Part model, mm, in its own coordinate system. Face numbers are marked on the shaded views. Round coordinates to 2 decimals unless told otherwise and drop trailing zeros. Loops run counter-clockwise (first coordinate to the right, second up) from the corner with the lowest first, then second, coordinate; pieces in that order, holes last. Notation, with made-up numbers: M -2,2.25 L 55,2.25 A11 cw 55,20.25 Z; hole C 25.25,78.25 d5. An arc over 180 degrees is marked long. Put each result on its own line as item: value. Start each with the question number.
1) Slice it at D-D on z = -4. Give the cut face in (x, y), then the cut area to 3 significant figures.
2) Probe line 1 along Y through (x, z) = (1.6, 0) (3 decimals); line 2 along Y through (x, z) = (1.9, -1.25) (3 decimals); line 3 along Z through (x, y) = (1.8, 1.75). List the from-to ranges inside material, lowest first.
3) Pull direction Z, two halves, no side cores. Call the marked faces 1, 2 and 3: +Z half, -Z half, draft (parallel to the pull), parting line (faces both ways), or undercut.
4) Slice it at A-A on z = 0. Give the cut face in (x, y) (3 decimals).
5) Slice it at B-B on x = 1.25. Give the cut face in (y, z) (3 decimals), then the cut area to 3 significant figures.
6) Drop a flat-ended pin along its axis: pin 1 Ø1 at (x, y) = (0.5, -3) entering from -Z. Give the stop position or say it passes through.
7) Slice it at C-C on y = 3. Give the cut face in (x, z), then the cut area to 3 significant figures.
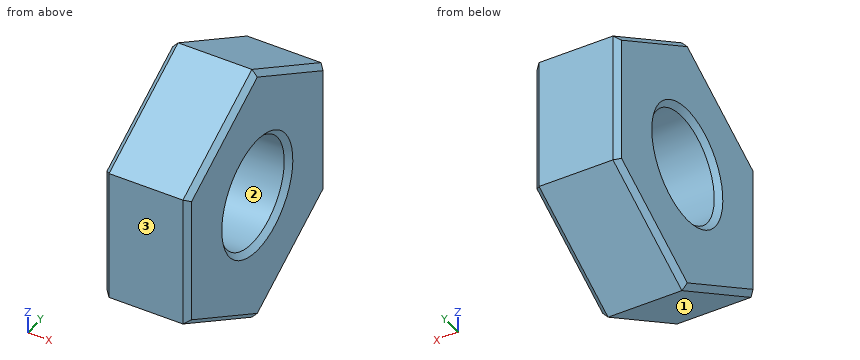
```python
from build123d import *

# Parameters (mm, degrees)
BOSS_EXTRUDE3_DEPTH = 3.15
SKETCH3_R           = 2
CUT_EXTRUDE2_DEPTH  = 7
CHAMFER1_SIZE       = 0.2


with BuildPart() as part:
    # Sketch2 → Boss-Extrude3 (new body)
    with BuildSketch(Plane(origin=(0, 0, 0), x_dir=(0, 0, -1), z_dir=(1, 0, 0))):
        Polygon((4.936344802, 0), (2.468172401, 4.275), (-2.468172401, 4.275), (-4.936344802, 0), (-2.468172401, -4.275), (2.468172401, -4.275), align=None)
    extrude(amount=BOSS_EXTRUDE3_DEPTH)

    # Sketch3 → Cut-Extrude2 (cut)
    with BuildSketch(Plane(origin=(3.15, 0, 0), x_dir=(0, 0, -1), z_dir=(1, 0, 0))):
        Circle(SKETCH3_R)
    extrude(amount=-CUT_EXTRUDE2_DEPTH, mode=Mode.SUBTRACT)

    # Chamfer1
    chamfer1_edges = [part.edges().sort_by_distance(p)[0] for p in [
        (3.15, 4.275, 0),
        (3.15, 2.1375, 3.702258601),
        (3.15, -2.1375, 3.702258601),
        (3.15, -4.275, 0),
        (0, 0, 2),
        (3.15, 0, 2),
        (3.15, -2.1375, -3.702258601),
        (0, -4.275, 0),
        (0, -2.1375, 3.702258601),
        (0, 2.1375, 3.702258601),
        (3.15, 2.1375, -3.702258601),
        (0, 4.275, 0),
        (0, 2.1375, -3.702258601),
        (0, -2.1375, -3.702258601),
    ]]
    chamfer(chamfer1_edges, length=CHAMFER1_SIZE)


solid = part.part
```
Recorded:
1. outline: M 0,-1.22 L 0.2,-1.62 L 2.95,-1.62 L 3.15,-1.22 L 3.15,1.22 L 2.95,1.62 L 0.2,1.62 L 0,1.22 Z
1. area: 10.1 mm2
2. line 1: y = -4.275 to -2, 2 to 4.275
2. line 2: y = -4.275 to -1.561, 1.561 to 4.275
2. line 3: z = -3.93 to -0.97, 0.97 to 3.93
3. face 1: -Z half
3. face 2: undercut
3. face 3: draft
4. outline: M 0,-4.075 L 0.2,-4.275 L 2.95,-4.275 L 3.15,-4.075 L 3.15,-2.2 L 2.95,-2 L 0.2,-2 L 0,-2.2 Z; M 0,2.2 L 0.2,2 L 2.95,2 L 3.15,2.2 L 3.15,4.075 L 2.95,4.275 L 0.2,4.275 L 0,4.075 Z
5. outline: M -4.275,-2.468 L 0,-4.936 L 4.275,-2.468 L 4.275,2.468 L 0,4.936 L -4.275,2.468 Z; hole C 0,0 d4
5. area: 50.7 mm2
6. pin 1: stops at z = -3.49
7. outline: M 0,-2.97 L 0.2,-3.2 L 2.95,-3.2 L 3.15,-2.97 L 3.15,2.97 L 2.95,3.2 L 0.2,3.2 L 0,2.97 Z
7. area: 20.1 mm2
